```python
from build123d import *

# Parameters (mm, degrees)
CUT_EXTRUDE_1_DEPTH = 2
CHAMFER_1_SIZE      = 0.5545
CHAMFER_1_SIZE2     = 0.320140724


with BuildPart() as part:
    # Эскиз1 → Повернуть1 (revolve)
    with BuildSketch(Plane(origin=(0, 0, 0), x_dir=(-1, 0, 0), z_dir=(0, 0, -1))):
        Polygon((-6, 2), (-6, 0), (0, 0), (0, 3), (-5, 3), align=None)
    revolve(axis=Axis((6, 0, 0), (-1, 0, 0)))

    # Эскиз2 → Вырез-Вытянуть1 (cut)
    with BuildSketch(Plane.ZY):
        Polygon((1.732050808, 0), (0.866025404, 1.5), (-0.866025404, 1.5), (-1.732050808, 0), (-0.866025404, -1.5), (0.866025404, -1.5), align=None)
    extrude(amount=-CUT_EXTRUDE_1_DEPTH, mode=Mode.SUBTRACT)

    # Фаска1
    chamfer_1_edges = [part.edges().sort_by_distance(p)[0] for p in [
        (0, -3, 0),
    ]]
    chamfer_1_side = [part.faces().sort_by_distance(p)[0] for p in [
        (0, -2.915147186, 0),
    ]]
    chamfer(chamfer_1_edges, length=CHAMFER_1_SIZE, length2=CHAMFER_1_SIZE2, reference=chamfer_1_side[0])


solid = part.part
```
Part model, mm, in its own coordinate system. A direction names the side the tool comes from. Round coordinates to 2 decimals unless told otherwise and drop trailing zeros. Write each loop counter-clockwise with the first axis right and the second up, starting at its lowest first coordinate (ties: lowest second). Pieces come first, ordered by that corner, then holes.
Item 1: Cut at A-A, the plane z = 0. Give the cut face in (x, y).
Results:
outline: (0, -2.45) - (0.32, -3) - (5, -3) - (6, -2) - (6, 2) - (5, 3) - (0.32, 3) - (0, 2.45) - (0, 1.5) - (2, 1.5) - (2, -1.5) - (0, -1.5) - close
Item 2: Probe L1, parallel to X at y = 0.65, z = -0.3; L2, parallel to Z at x = 1.4, y = 0.55; L3, parallel to X at y = 1.6, z = -2.25. List the from-to ranges inside material, lowest first.
Results:
L1: x = 2 to 6
L2: z = -2.95 to -1.41, 1.41 to 2.95
L3: x = 0.18 to 5.24
Item 3: Drop flat-ended pins along their axis: pin 1 Ø2.5 at (y, z) = (-0.5, 0.5) entering from -X; pin 2 Ø1.5 at (x, z) = (4.5, 1.5) entering from +Y; pin 3 Ø1 at (x, z) = (4, -1.5) entering from +Y. Give the stop position or say it passes through.
Results:
pin 1: stops at x = 0
pin 2: stops at y = 2.9
pin 3: stops at y = 2.83
Item 4: Cut at B-B, the plane x = 1.15. Give the cut face in (y, z), plus the area to 3 significant figures.
Results:
outline: circle Ø6 at (0, 0); hole (-1.5, -0.87) - (0, -1.73) - (1.5, -0.87) - (1.5, 0.87) - (0, 1.73) - (-1.5, 0.87) - close
area: 20.5 mm2
Item 5: Cut at C-C, the plane x = 2.9. Give the cut face in (y, z), plus the area to 3 significant figures.
Results:
outline: circle Ø6 at (0, 0)
area: 28.3 mm2
Item 6: Which spindle directions (+Z, -Z, +X, -X, +Y, -Y) get a long thin tool onto all of the face, cutting with end or side? Do faces 1 (the flat face through (6, 0, 0)), 2 (the flat face through (2, 0, 0)). Say none if no direction does.
Results:
face 1: +Z, -Z, +X, +Y, -Y
face 2: -X
Item 7: Two-plate mould, pull along Y, no slides. Class faces 3 (the cylindrical face through (3, -3, 0)), 4 (the flat face through (0, -2, 0)), 5 (the flat face through (0.986, 0.76, -1.293)), 6 (the flat face through (0.986, 0.74, 1.305)): +Y half, -Y half, draft (parallel to the pull), parting line (faces both ways), or undercut.
Results:
face 3: parting line
face 4: draft
face 5: undercut
face 6: undercut
